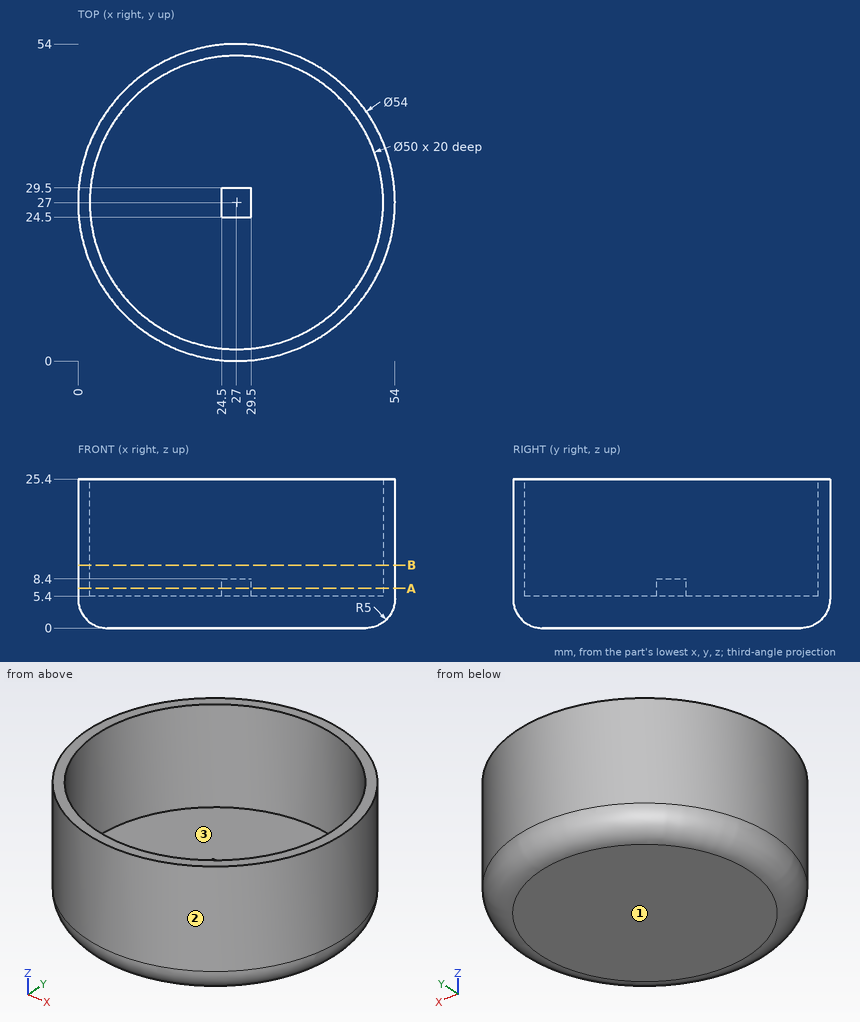
Part print with two shaded views. Sizes in mm from the minimum x, y, z corner. Coordinates: 2 decimals unless noted, no trailing zeros. Order: outer loops, then holes, each group sorted by start corner. A loop starts at its lowest first (then second) coordinate and runs counter-clockwise, first axis right, second up.
(1) Mould opens along Y. For the marked faces 1, 2 and 3 say: released by +Y, released by -Y, zero draft, split by the parting line, or undercut.
Solution:
face 1: zero draft
face 2: split by the parting line
face 3: undercut
(2) Saw through at A-A, the plane z = 6.75. Write the cut outline in (x, y), and give its area (3 significant figures).
Solution:
outline: circle Ø54 at (27, 27); (24.5, 24.5) - (29.5, 24.5) - (29.5, 29.5) - (24.5, 29.5) - close; hole circle Ø50 at (27, 27)
area: 352 mm2
(3) Saw through at B-B, the plane z = 10.75. Write the cut outline in (x, y).
Solution:
outline: circle Ø54 at (27, 27); hole circle Ø50 at (27, 27)
(4) Drill centre lines: L1, parallel to Y at x = 27, z = 17.75; L2, parallel to Z at x = 15.5, y = 24.5; L3, parallel to Y at x = 12, z = 8.25. Where is each one in solid material? Low to high.
Solution:
L1: y = 0 to 2, 52 to 54
L2: z = 0 to 5.4
L3: y = 4.55 to 7, 47 to 49.45
(5) Pin check, flat tips, straight feed: pin 1 Ø4 at (x, y) = (28, 28) entering from +Z; pin 2 Ø2.5 at (x, z) = (27.5, 7.5) entering from +Y; pin 3 Ø2 at (x, z) = (42.5, 18.5) entering from -Y. Stop position of each tip, or through.
Solution:
pin 1: stops at z = 8.4
pin 2: stops at y = 54
pin 3: stops at y = 4.22
